from build123d import *

# Parameters (mm, degrees)
TUBE_SQUARE_TS3X3X0_3125_1_DEPTH = 1615
M20X2_5_TAPPED_HOLE1_D           = 17.5
SKETCH19_R                       = 5
CUT_EXTRUDE1_DEPTH               = 838.470148722


with BuildPart() as part:
    # Sketch14 → Tube square TS3X3X0.3125(1) (new body)
    with BuildSketch(Plane(origin=(0, 0, -807.5), x_dir=(0, -1, 0), z_dir=(0, 0, 1))):
        with BuildLine():
            Line((-118, -90), (118, -90))
            ThreePointArc((118, -90), (126.485281374, -86.485281374), (130, -78))
            Line((130, -78), (130, 78))
            ThreePointArc((130, 78), (126.485281374, 86.485281374), (118, 90))
            Line((118, 90), (-118, 90))
            ThreePointArc((-118, 90), (-126.485281374, 86.485281374), (-130, 78))
            Line((-130, 78), (-130, -78))
            ThreePointArc((-130, -78), (-126.485281374, -86.485281374), (-118, -90))
        make_face()
        with BuildLine():
            Line((-118, -80), (118, -80))
            ThreePointArc((118, -80), (119.414213562, -79.414213562), (120, -78))
            Line((120, -78), (120, 78))
            ThreePointArc((120, 78), (119.414213562, 79.414213562), (118, 80))
            Line((118, 80), (-118, 80))
            ThreePointArc((-118, 80), (-119.414213562, 79.414213562), (-120, 78))
            Line((-120, 78), (-120, -78))
            ThreePointArc((-120, -78), (-119.414213562, -79.414213562), (-118, -80))
        make_face(mode=Mode.SUBTRACT)
    extrude(amount=TUBE_SQUARE_TS3X3X0_3125_1_DEPTH)

    # M20x2.5 Tapped Hole1 (through all)
    with Locations(Plane(origin=(90, 0, 0), x_dir=(0, 0, -1), z_dir=(1, 0, 0))):
        with Locations((717.5, 30), (557.5, 30), (557.5, -30), (717.5, -30)):
            Hole(M20X2_5_TAPPED_HOLE1_D / 2)

    # Sketch19 → Cut-Extrude1 (cut, through all)
    with BuildSketch(Plane(origin=(90, 0, 0), x_dir=(0, 0, -1), z_dir=(1, 0, 0))):
        with Locations(Location((-642.5, 0, 0), (0, 0, 90))):
            Circle(SKETCH19_R)
    extrude(amount=-CUT_EXTRUDE1_DEPTH, mode=Mode.SUBTRACT)


solid = part.part
Check sheet for the modelled part. Datum: model origin and axes. Units: mm. A direction names the side the tool comes from. Coordinates: 2 decimals unless noted, no trailing zeros. Write each loop counter-clockwise with the first axis right and the second up, starting at its lowest first coordinate (ties: lowest second). Pieces come first, ordered by that corner, then holes.
Item 1: Cross-section at C-C on z = -63.5. Record the boundary of the cut face in (x, y), then the cut area to 3 significant figures.
Numbers:
outline: (-90, -118) arc R12 ccw to (-78, -130) - (78, -130) arc R12 ccw to (90, -118) - (90, 118) arc R12 ccw to (78, 130) - (-78, 130) arc R12 ccw to (-90, 118) - close; hole (-80, -118) arc R2 ccw to (-78, -120) - (78, -120) arc R2 ccw to (80, -118) - (80, 118) arc R2 ccw to (78, 120) - (-78, 120) arc R2 ccw to (-80, 118) - close
area: 8,280 mm2
Item 2: Cross-section at B-B on x = -11.5. Record the boundary of the cut face in (y, z).
Numbers:
outline: (-130, -807.5) - (-120, -807.5) - (-120, 807.5) - (-130, 807.5) - close; (120, -807.5) - (130, -807.5) - (130, 807.5) - (120, 807.5) - close
Item 3: Mould release check, pull along X, two halves, no side actions. Record for faces 1 (the face through (80, -2, -11)), 2 (the face through (-80, 2, -11)), 3 (the face through (80.4, 0.6, -807.5)), 4 (the face through (90, -2, -11)): released by +X, released by -X, zero draft, split by the parting line, or undercut.
Numbers:
face 1: undercut
face 2: undercut
face 3: zero draft
face 4: released by +X
Item 4: Scan lines: probe 1 along Y at (x, z) = (44.5, -49); probe 2 along X at (y, z) = (-56.5, 92); probe 3 along Z at (x, y) = (-87, 0). Record each from-to range of solid material in increasing order.
Numbers:
probe 1: y = -130 to -120, 120 to 130
probe 2: x = -90 to -80, 80 to 90
probe 3: z = -807.5 to 637.5, 647.5 to 807.5
Item 5: Access from +Z, -Z, +X, -X, +Y, -Y to the whole of each face (thin tool, end or side, straight path). Record for faces 5 (the face through (-1, -120, -11)), 6 (the face through (-90, 2, -11)).
Numbers:
face 5: +Z, -Z
face 6: +Z, -Z, -X, +Y, -Y
Item 6: Depth check by flat-ended pin: pin 1 Ø10.5 at (y, z) = (-30, -717.5) entering from +X. Enter the tip coordinate at first touch or a pass-through.
Numbers:
pin 1: passes through
Item 7: Cross-section at A-A on y = 102. Record the boundary of the cut face in (x, z), then the cut area to 3 significant figures.
Numbers:
outline: (-90, -807.5) - (-80, -807.5) - (-80, 807.5) - (-90, 807.5) - close; (80, -807.5) - (90, -807.5) - (90, 807.5) - (80, 807.5) - close
area: 32,300 mm2
